Part print with two shaded views. Sizes in mm from the minimum x, y, z corner. A direction names the side the tool comes from. Round coordinates to 2 decimals unless told otherwise and drop trailing zeros. Order: outer loops, then holes, each group sorted by start corner. A loop starts at its lowest first (then second) coordinate and runs counter-clockwise, first axis right, second up. Notation, with made-up numbers: M -18.5,50 L 22.5,50 A19 ccw 22.5,58 Z; hole C -19,41 d6. An arc over 180 degrees is marked long. Answer as a JSON object with one key per item and string values.
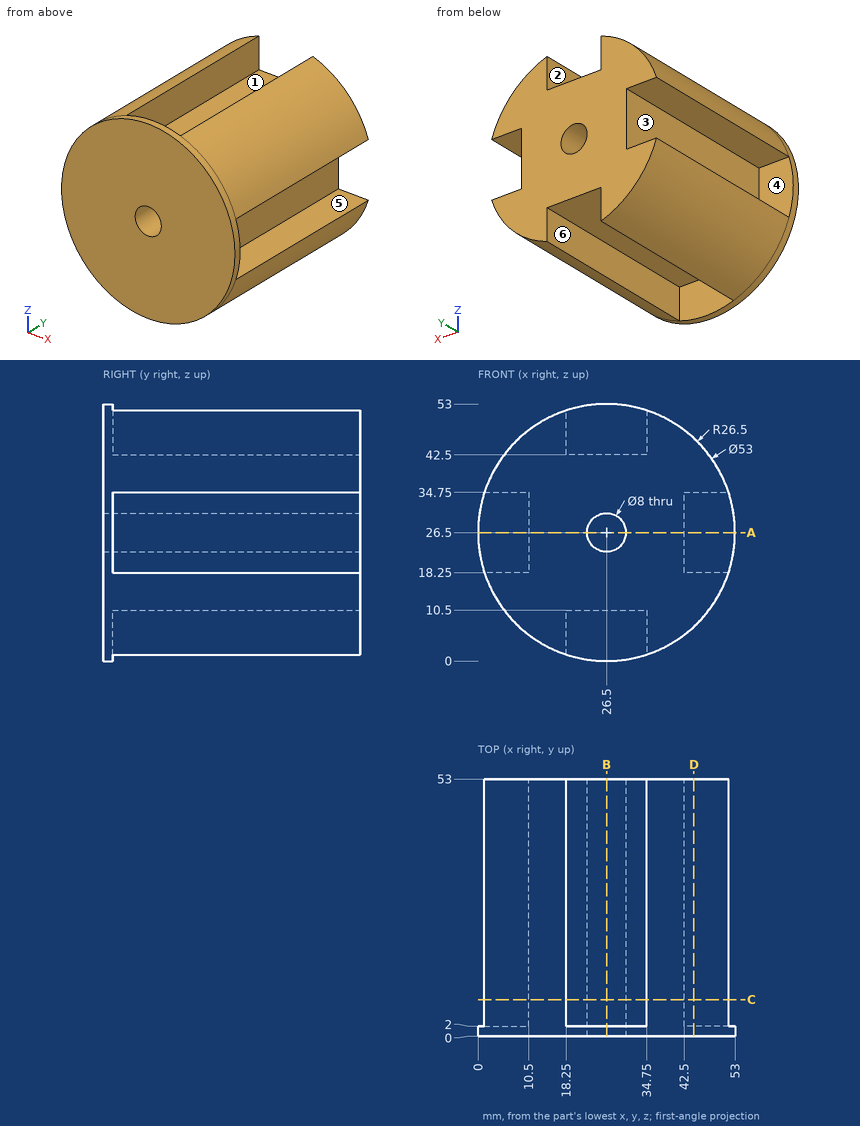
Item 1: Saw through at B-B on x = 26.5. List the corners of the cut face in (y, z), and give its area (3 significant figures).
Worked answers:
{"outline": "M 0,0 L 2,0 L 2,10.5 L 53,10.5 L 53,22.5 L 0,22.5 Z; M 0,30.5 L 53,30.5 L 53,42.5 L 2,42.5 L 2,53 L 0,53 Z", "area": "1,310 mm2"}
Item 2: Saw through at D-D on x = 44.5. List the corners of the cut face in (y, z).
Worked answers:
{"outline": "M 0,7.05 L 53,7.05 L 53,18.25 L 2,18.25 L 2,34.75 L 53,34.75 L 53,45.95 L 0,45.95 Z"}
Item 3: Drop flat-ended pins along their axis: pin 1 Ø12 at (y, z) = (10, 28) entering from +X; pin 2 Ø10 at (y, z) = (17.5, 45.5) entering from +X; pin 3 Ø3 at (x, y) = (8, 21.5) entering from -Z; pin 4 Ø9 at (x, z) = (26.5, 26.5) entering from -Y. Give the stop position or say it passes through.
Worked answers:
{"pin 1": "stops at x = 42.5", "pin 2": "stops at x = 49", "pin 3": "stops at z = 6.17", "pin 4": "stops at y = 0"}
Item 4: Two-plate mould, pull along Z, no slides. Class the marked faces 1, 2 and 3: released by +Z, released by -Z, zero draft, split by the parting line, or undercut.
Worked answers:
{"face 1": "released by +Z", "face 2": "zero draft", "face 3": "undercut"}
Item 5: Wall check: line 1 along Z through (x, y) = (26.5, 15); line 2 along Y through (x, z) = (48, 21.5). Give the ranges that are in metal, low to high. Write a range as [from, to].
Worked answers:
{"line 1": "z = [10.5, 22.5], [30.5, 42.5]", "line 2": "y = [0, 2]"}
Item 6: Saw through at C-C on y = 7.5. List the corners of the cut face in (x, z), and give its area (3 significant figures).
Worked answers:
{"outline": "M 1.32,18.25 A26.5 ccw 18.25,1.32 L 18.25,10.5 L 34.75,10.5 L 34.75,1.32 A26.5 ccw 51.68,18.25 L 42.5,18.25 L 42.5,34.75 L 51.68,34.75 A26.5 ccw 34.75,51.68 L 34.75,42.5 L 18.25,42.5 L 18.25,51.68 A26.5 ccw 1.32,34.75 L 10.5,34.75 L 10.5,18.25 Z; hole C 26.5,26.5 d8", "area": "1,490 mm2"}
Item 7: 3-axis set-ups, long thin cutter, end or side, ignore diameter. For the marked faces 4, 5 and 6: which of +Z, -Z, +X, -X, +Y, -Y reach the whole face in a straight line?
Worked answers:
{"face 4": "-X, +Y", "face 5": "+X, +Y", "face 6": "-Z, +Y"}
Item 8: Saw through at A-A on z = 26.5. List the corners of the cut face in (x, y).
Worked answers:
{"outline": "M 0,0 L 22.5,0 L 22.5,53 L 10.5,53 L 10.5,2 L 0,2 Z; M 30.5,0 L 53,0 L 53,2 L 42.5,2 L 42.5,53 L 30.5,53 Z"}
